```python
from build123d import *

# Parameters (mm, degrees)
F0_W     = 50
F0_H     = 9
F0_R     = 4.5
F1_DEPTH = 3


with BuildPart() as f1:
    # F0 (on Top) → F1 (new body)
    with BuildSketch(Plane.XY):
        with BuildLine():
            ThreePointArc((0, -5), (-1.464466, -1.464466), (-5, 0))
            Line((-5, 0), (-50, 0))
            Line((-50, 0), (-550, 0))
            Line((-550, 0), (-595, 0))
            ThreePointArc((-595, 0), (-598.535534, -1.464466), (-600, -5))
            Line((-600, -5), (-600, -95))
            ThreePointArc((-600, -95), (-598.535534, -98.535534), (-595, -100))
            Line((-595, -100), (-550, -100))
            Line((-550, -100), (-50, -100))
            Line((-50, -100), (-5, -100))
            ThreePointArc((-5, -100), (-1.464466, -98.535534), (0, -95))
            Line((0, -95), (0, -5))
        make_face()
        with Locations((-535, -75.006462)):
            Rectangle(F0_W, F0_H, mode=Mode.SUBTRACT)
        with Locations((-575, -75)):
            Circle(F0_R, mode=Mode.SUBTRACT)
        with Locations((-65, -75.006462)):
            Rectangle(F0_W, F0_H, mode=Mode.SUBTRACT)
        with Locations((-25, -75)):
            Circle(F0_R, mode=Mode.SUBTRACT)
        with Locations((-575, -25)):
            Circle(F0_R, mode=Mode.SUBTRACT)
        with Locations((-535, -24.993538)):
            Rectangle(F0_W, F0_H, mode=Mode.SUBTRACT)
        with Locations((-65, -24.993538)):
            Rectangle(F0_W, F0_H, mode=Mode.SUBTRACT)
        with Locations((-25, -25)):
            Circle(F0_R, mode=Mode.SUBTRACT)
    extrude(amount=F1_DEPTH)


solid = f1.part
```
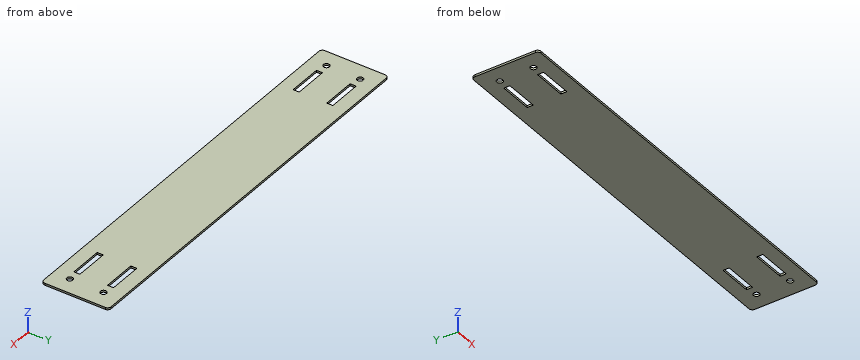
Part model, mm, in its own coordinate system. Round coordinates to 2 decimals unless told otherwise and drop trailing zeros. Loops run counter-clockwise (first coordinate to the right, second up) from the corner with the lowest first, then second, coordinate; pieces in that order, holes last.
1. Drill centre lines: line 1 along X through (y, z) = (-76, 2.5); line 2 along Y through (x, z) = (-575, 0.95). Where is each one in solid material? Low to high.
Solutions:
line 1: x = -600 to -579.39, -570.61 to -560, -510 to -90, -40 to -29.39, -20.61 to 0
line 2: y = -100 to -79.5, -70.5 to -29.5, -20.5 to 0
2. Slice it at A-A (x = -58). Give the cut face in (y, z).
Solutions:
outline: (-100, 0) - (-79.51, 0) - (-79.51, 3) - (-100, 3) - close; (-70.51, 0) - (-29.49, 0) - (-29.49, 3) - (-70.51, 3) - close; (-20.49, 0) - (0, 0) - (0, 3) - (-20.49, 3) - close
3. Flat gauge pin, fed straight in: pin 1 (10.5 mm diameter, centred on x = -575, y = -25, fed in from +Z). Where does the tip first touch, or does it go through?
Solutions:
pin 1: stops at z = 3
4. Slice it at B-B (z = 1.8). Count the separate pieces of the cut face and the enclosed holes in it, and give its area (3 significant figures).
Solutions:
separate pieces: 1
enclosed holes: 8
area: 57,900 mm2
